Can you work these out from the drawing? Everything is in mm from the part's minimum corner. Give positions to 0.01 mm unless a question says otherwise; leave off trailing zeros. Order: outer loops, then holes, each group sorted by start corner. A loop starts at its lowest first (then second) coordinate and runs counter-clockwise, first axis right, second up. Notation, with made-up numbers: M 82,69.25 L 99,69.25 A26 ccw 99,87.25 Z; hole C 63.5,-3 d10. An arc over 180 degrees is marked long. Use a Markdown table: item, result. Add a question column.
Item 1: Suppose I cut it at A-A on x = 0.9. Write out the boundary of the cut face in (y, z).
Item 2: If we mould it in two halves opening along Z, with no side actions, what happens to the marked faces 1, 2, 3 and 4? For each: released by +Z, released by -Z, zero draft, split by the parting line, or undercut.
Item 3: I'm going to push a flat-ended pin straight in: pin 1 Ø1.9 at (y, z) = (4.95, 4.95) entering from -X. Where does the tip first touch, or does it pass through?
Item 4: If I drill on L1, parallel to Z at x = 0.8, y = 5; L2, parallel to Y at x = 1.3, z = 4.75; L3, parallel to Z at x = 0.7, y = 2, over which ranges is the centre line in solid material (lowest first)? Write a range as from..to.
Item 5: Suppose I cut it at C-C on y = 1.75. Write out the boundary of the cut face in (x, z).
Item 6: Suppose I cut it at B-B on y = 9. Write out the boundary of the cut face in (x, z).
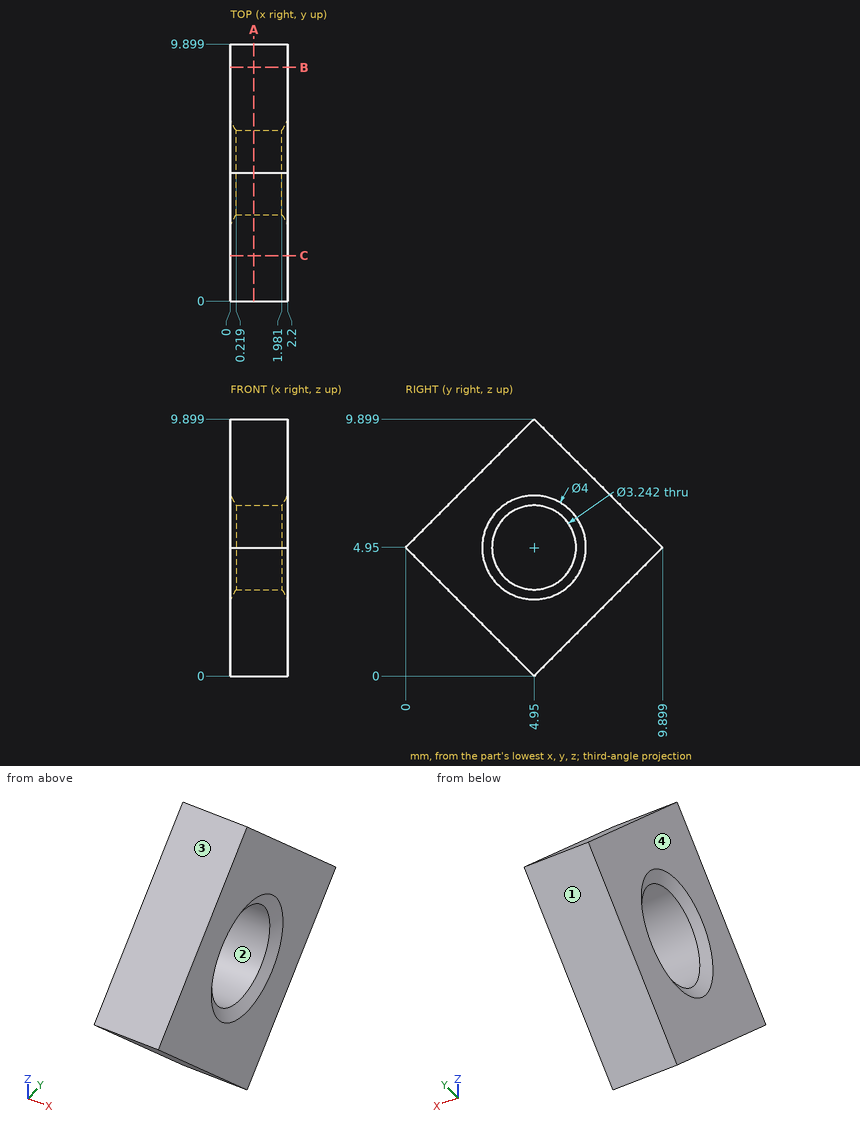
Findings below:
| question | item | result |
|---|---|---|
| 1 | outline | M 0,4.95 L 4.95,0 L 9.9,4.95 L 4.95,9.9 Z; hole C 4.95,4.95 d3.24 |
| 2 | face 1 | released by -Z |
| 2 | face 2 | undercut |
| 2 | face 3 | released by +Z |
| 2 | face 4 | zero draft |
| 3 | pin 1 | passes through |
| 4 | L1 | z = 0.05..3.33, 6.57..9.85 |
| 4 | L2 | y = 0.2..3.34, 6.56..9.7 |
| 4 | L3 | z = 2.95..6.95 |
| 5 | outline | M 0,3.2 L 2.2,3.2 L 2.2,6.7 L 0,6.7 Z |
| 6 | outline | M 0,4.05 L 2.2,4.05 L 2.2,5.85 L 0,5.85 Z |
